Geometry check sheet. Reference: the model listing, model coordinates, mm. A direction names the side the tool comes from. Round coordinates to 2 decimals unless told otherwise and drop trailing zeros. Loops run counter-clockwise (first coordinate to the right, second up) from the corner with the lowest first, then second, coordinate; pieces in that order, holes last.
```python
from build123d import *

# Parameters (mm, degrees)
SKETCH1_W           = 35.4
SKETCH1_H           = 40.2
BOSS_EXTRUDE1_DEPTH = 7
SKETCH2_W           = 29
SKETCH2_H           = 6
CUT_EXTRUDE1_DEPTH  = 29.8
SKETCH3_R           = 1.25
CUT_EXTRUDE2_DEPTH  = 28.682124196
SKETCH4_W           = 10
SKETCH4_H           = 5
BOSS_EXTRUDE2_DEPTH = 4.7625
CHAMFER1_SIZE       = 5.1
CHAMFER1_SIZE2      = 6
MIRROR4_START       = -26.778357323
MIRROR4_OUTLINE_W   = 11
MIRROR4_OUTLINE_H   = 9
MIRROR4_DEPTH       = 3.885890521
FILLET1_R           = 1


# Read off the part's stored shape, not the designer's step: Mirror4
with BuildPart() as part:
    # Sketch1 → Boss-Extrude1 (new body)
    with BuildSketch(Plane(origin=(0, 0, 0), x_dir=(1, 0, 0), z_dir=(0, 1, 0))):
        Rectangle(SKETCH1_W, SKETCH1_H)
    extrude(amount=BOSS_EXTRUDE1_DEPTH)

    # Sketch2 → Cut-Extrude1 (cut)
    with BuildSketch(Plane(origin=(17.7, 0, 0), x_dir=(0, 0, -1), z_dir=(1, 0, 0))):
        with Locations((0, 3)):
            Rectangle(SKETCH2_W, SKETCH2_H)
    extrude(amount=-CUT_EXTRUDE1_DEPTH, mode=Mode.SUBTRACT)

    # Sketch3 → Cut-Extrude2 (cut, through all)
    with BuildSketch(Plane(origin=(0, 7, 0), x_dir=(1, 0, 0), z_dir=(0, 1, 0))):
        with Locations(Location((14.9, 17.3, 0), (0, 0, 270))):
            Circle(SKETCH3_R)
        with Locations(Location((-7.1, 17.3, 0), (0, 0, 270))):
            Circle(SKETCH3_R)
        with Locations(Location((-14.9, 11, 0), (0, 0, 270))):
            Circle(SKETCH3_R)
    cut_extrude2 = extrude(amount=-CUT_EXTRUDE2_DEPTH, mode=Mode.SUBTRACT)

    # Sketch4 → Boss-Extrude2 (add)
    with BuildSketch(Plane(origin=(0, 7, 0), x_dir=(-1, 0, 0), z_dir=(0, 1, 0))):
        with Locations((4.7, -9.6)):
            Rectangle(SKETCH4_W, SKETCH4_H)
    boss_extrude2 = extrude(amount=BOSS_EXTRUDE2_DEPTH)

    # Mirror1: Cut-Extrude2, Boss-Extrude2 across plane
    add(cut_extrude2.mirror(Plane.XY), mode=Mode.SUBTRACT)
    add(boss_extrude2.mirror(Plane.XY))

    # Chamfer1
    chamfer1_edges = [part.edges().sort_by_distance(p)[0] for p in [
        (-17.7, 3.5, 20.1),
    ]]
    chamfer1_side = [part.faces().sort_by_distance(p)[0] for p in [
        (-17.7, 3.5, 0),
    ]]
    chamfer(chamfer1_edges, length=CHAMFER1_SIZE, length2=CHAMFER1_SIZE2, reference=chamfer1_side[0])

    # Mirror4 outline → Mirror4 (cut)
    with BuildSketch(Plane(origin=(0, 0, 0), x_dir=(0.7619393177594598, 0, -0.6476484200955399), z_dir=(0.6476484200955399, 0, 0.7619393177594598)).offset(MIRROR4_START)):
        with Locations((0.5, 3.5)):
            Rectangle(MIRROR4_OUTLINE_W, MIRROR4_OUTLINE_H)
    extrude(amount=MIRROR4_DEPTH, mode=Mode.SUBTRACT)

    # Fillet1
    fillet1_edges = [part.edges().sort_by_distance(p)[0] for p in [
        (17.7, 7, 0),
        (0.3, 9.38125, -7.1),
        (0.3, 9.38125, -12.1),
        (-9.7, 9.38125, -12.1),
        (-9.7, 9.38125, -7.1),
        (0.3, 11.7625, -9.6),
        (-4.7, 11.7625, -12.1),
        (-9.7, 11.7625, -9.6),
        (-4.7, 11.7625, -7.1),
        (0.3, 11.7625, 9.6),
        (0.3, 9.38125, 12.1),
        (-4.7, 11.7625, 7.1),
        (0.3, 9.38125, 7.1),
        (-9.7, 11.7625, 9.6),
        (-9.7, 9.38125, 7.1),
        (-4.7, 11.7625, 12.1),
        (-9.7, 9.38125, 12.1),
        (3, 7, -20.1),
        (17.7, 3.5, 20.1),
        (17.7, 3.5, -20.1),
        (3, 7, 20.1),
        (-11.7, 3.5, 20.1),
        (-17.7, 3.5, 15),
        (-14.7, 7, 17.55),
        (-17.7, 7, 0),
        (-11.7, 3.5, -20.1),
        (-17.7, 3.5, -15),
        (-14.7, 7, -17.55),
    ]]
    fillet(fillet1_edges, radius=FILLET1_R - 0.0001)  # a hair under: the kernel refuses the full size


solid = part.part
```
1) Scan lines: line 1 along Z through (x, y) = (-1, 1.75); line 2 along X through (y, z) = (3.75, -11); line 3 along X through (y, z) = (3.75, -17.3). Record each from-to range of solid material in increasing order.
Report:
line 1: z = -20.1 to -14.5, 14.5 to 20.1
line 2: x = -17.7 to -16.15, -13.65 to -12.1
line 3: x = -14.99 to -8.35, -5.85 to 13.65, 16.15 to 17.7
2) Mould release check, pull along X, two halves, no side actions. Record for faces 1 (the face through (-6.72, 3.55, -16.11)), 2 (the face through (3, 3, 14.5)), 3 (the face through (17.415, 3.042, 19.799)), 4 (the face through (-15.66, 3.55, -11.99)): +X half, -X half, draft (parallel to the pull), parting line (faces both ways), or undercut.
Report:
face 1: undercut
face 2: draft
face 3: +X half
face 4: undercut
3) Access from +Z, -Z, +X, -X, +Y, -Y to the whole of each face (thin tool, end or side, straight path). Record for faces 5 (the face through (-9.399, 8.908, 11.815)), 6 (the face through (-9.7, 9, -10)), 7 (the face through (-9.415, 8.908, -7.401)), 8 (the face through (-5, 9, -12.1)), 9 (the face through (-9.399, 8.908, -11.815)).
Report:
face 5: +Z, -X, +Y
face 6: +Z, -Z, -X, +Y
face 7: -X, +Y
face 8: -Z, +X, -X, +Y
face 9: -Z, -X, +Y
4) Sectioned sample at C-C, the plane x = -1.5. Record the cut outline in (y, z), then the cut area to 3 significant figures.
Report:
outline: (0, -20.1) - (6, -20.1) arc R1 ccw to (7, -19.1) - (7, -12.1) - (10.76, -12.1) arc R1 ccw to (11.76, -11.1) - (11.76, -8.1) arc R1 ccw to (10.76, -7.1) - (7, -7.1) - (7, 7.1) - (10.76, 7.1) arc R1 ccw to (11.76, 8.1) - (11.76, 11.1) arc R1 ccw to (10.76, 12.1) - (7, 12.1) - (7, 19.1) arc R1 ccw to (6, 20.1) - (0, 20.1) - (0, 14.5) - (6, 14.5) - (6, -14.5) - (0, -14.5) - close
area: 154 mm2
5) Sectioned sample at A-A, the plane x = 14.9. Record the cut outline in (y, z).
Report:
outline: (0, -20.1) - (6, -20.1) arc R1 ccw to (7, -19.1) - (7, -18.55) - (0, -18.55) - close; (0, -16.05) - (7, -16.05) - (7, 16.05) - (0, 16.05) - (0, 14.5) - (6, 14.5) - (6, -14.5) - (0, -14.5) - close; (0, 18.55) - (7, 18.55) - (7, 19.1) arc R1 ccw to (6, 20.1) - (0, 20.1) - close
6) Gauge pin test, flat ends, axial feed: pin 1 (2.5 mm diameter, centred on y = 8, z = -10, fed in from +X); pin 2 (3 mm diameter, centred on y = 3, z = -5, fed in from +X); pin 3 (4 mm diameter, centred on x = -14.9, z = -11, fed in from +Y); pin 4 (4 mm diameter, centred on x = 14.9, z = -17.3, fed in from -Y). Record the tip position at first contact, or that the pin passes through.
Report:
pin 1: stops at x = 17.36
pin 2: stops at x = -12.1
pin 3: stops at y = 7
pin 4: stops at y = 0
